Source: three-view drawing plus pictorial views. Frame: mm from the lowest corner of the part. Coordinates: 2 decimals unless noted, no trailing zeros. Write each loop counter-clockwise with the first axis right and the second up, starting at its lowest first coordinate (ties: lowest second). Pieces come first, ordered by that corner, then holes. Notation, with made-up numbers: (7.5, 74.5) - (23.5, 74.5) arc R22 cw to (23.5, 93.5) - close; hole circle Ø8 at (-32.75, 24.25). An arc over 180 degrees is marked (long way). Answer as a JSON object with one key per item and string values. Group by question number.
Item 1: Line query: line 1 along Z through (x, y) = (51.5, 1.3); line 2 along X through (y, z) = (1.95, 29) (1 decimal); line 3 along Z through (x, y) = (50.5, 0.3). Output: solid intervals per line, ascending. Write a range as from..to.
Item 2: Section C-C on x = 6.5. Return loops of the section in (y, z) (3 decimals), and give its area (3 significant figures).
Item 3: First-contact query: pin 1 Ø2.5 at (x, z) = (51.5, 6.5) entering from +Y; pin 2 Ø1 at (x, y) = (92.5, 2) entering from +Z; pin 3 Ø0.9 at (y, z) = (1, 53.5) entering from -X; pin 4 Ø0.9 at (x, y) = (49.5, 2) entering from +Z. Flat tips, straight axial feed; report the tip coordinate or a pass-through.
Item 4: Mould query, pull axis Y, two halves, no side actions, for the marked faces 1 and 2. Classes: pulls with the +Y half, pulls with the -Y half, needs draft (parallel to the pull), parting line crosses it, or undercut.
Item 5: Section D-D on z = 96.5. Return loops of the section in (x, y) (3 decimals).
Item 6: Section A-A on z = 51.5. Return loops of the section in (x, y).
Item 7: Section B-B on x = 51.5. Return loops of the section in (y, z).
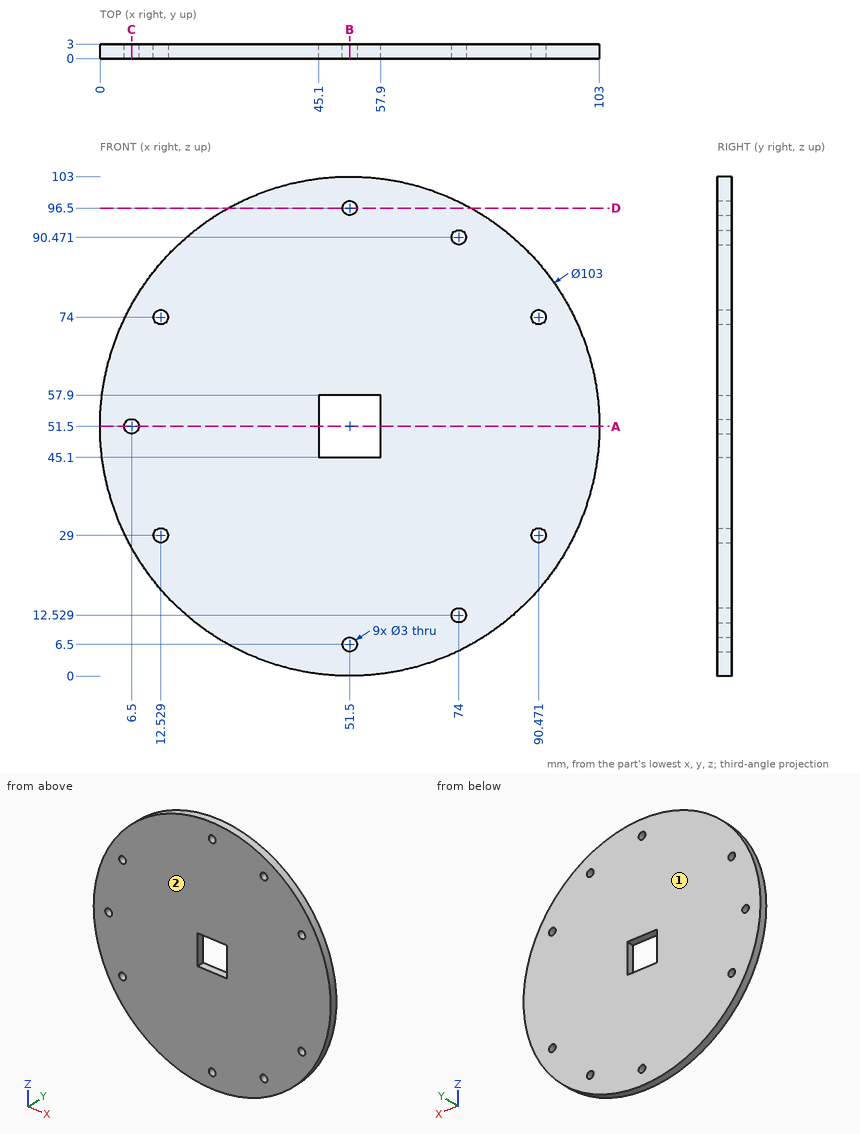
Checks:
{
 "1": {"line 1": "0..5, 8..45.1, 57.9..95, 98..103", "line 2": "5.2..11, 14..89, 92..97.8", "line 3": "0.01..5.38, 7.62..45.1, 57.9..95.38, 97.62..102.99"},
 "2": {"outline": "(0, 26.455) - (3, 26.455) - (3, 50) - (0, 50) - close; (0, 53) - (3, 53) - (3, 76.545) - (0, 76.545) - close", "area": "141 mm^2"},
 "3": {"pin 1": "through", "pin 2": "z = 83.31", "pin 3": "x = 0.02", "pin 4": "z = 102.98"},
 "4": {"face 1": "pulls with the +Y half", "face 2": "pulls with the -Y half"},
 "5": {"outline": "(26.455, 0) - (50, 0) - (50, 3) - (26.455, 3) - close; (53, 0) - (76.545, 0) - (76.545, 3) - (53, 3) - close"},
 "6": {"outline": "(0, 0) - (5, 0) - (5, 3) - (0, 3) - close; (8, 0) - (45.1, 0) - (45.1, 3) - (8, 3) - close; (57.9, 0) - (103, 0) - (103, 3) - (57.9, 3) - close"},
 "7": {"outline": "(0, 0) - (3, 0) - (3, 5) - (0, 5) - close; (0, 8) - (3, 8) - (3, 45.1) - (0, 45.1) - close; (0, 57.9) - (3, 57.9) - (3, 95) - (0, 95) - close; (0, 98) - (3, 98) - (3, 103) - (0, 103) - close"}
}
